Source: three-view drawing plus pictorial views. Frame: mm from the lowest corner of the part. Give positions to 0.01 mm unless a question says otherwise; leave off trailing zeros. Order: outer loops, then holes, each group sorted by start corner. A loop starts at its lowest first (then second) coordinate and runs counter-clockwise, first axis right, second up.
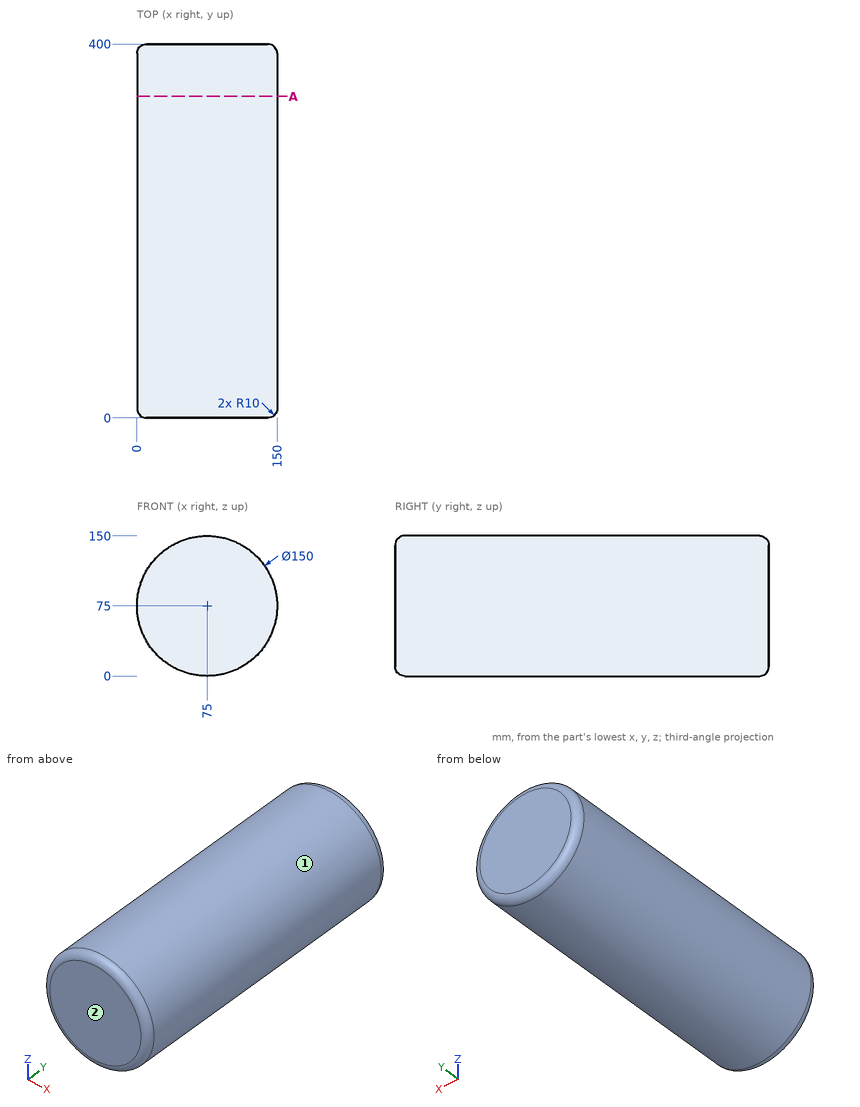
1) Pull-direction query (Z, two-part tool) for the marked faces 1 and 2; classes: +Z half, -Z half, draft (parallel to the pull), parting line (faces both ways), or undercut.
Checks:
face 1: parting line
face 2: draft
2) First-contact query: pin 1 Ø1 at (y, z) = (55.5, 70.5) entering from +X; pin 2 Ø5 at (x, y) = (35, 307) entering from +Z; pin 3 Ø8 at (y, z) = (84, 64.5) entering from -X. Flat tips, straight axial feed; report the tip coordinate or a pass-through.
Checks:
pin 1: stops at x = 149.89
pin 2: stops at z = 139.95
pin 3: stops at x = 0.28
3) Ray query, L1, parallel to X at y = 24, z = 71.5; L2, parallel to Z at x = 78, y = 77.5; L3, parallel to X at y = 313, z = 39.5. Return the intervals inside material, ascending.
Checks:
L1: x = 0.08 to 149.92
L2: z = 0.06 to 149.94
L3: x = 8.93 to 141.07
4) Section query A-A on y = 344. Output: boundary loops of the cut face in (x, z), and give its area (3 significant figures).
Checks:
outline: circle Ø150 at (75, 75)
area: 17,700 mm2
